```python
from build123d import *

# Parameters (mm, degrees)
SKETCH1_W                = 42.4
SKETCH1_H                = 42.4
BOSS_EXTRUDE1_DEPTH      = 5
BOSS_EXTRUDE2_DEPTH      = 5
BOSS_EXTRUDE2_DEPTH_BACK = 5
SKETCH3_W                = 2.630753666
SKETCH3_H                = 21.2
SKETCH3_W_2              = 21.2
SKETCH3_H_2              = 2.630753666
BOSS_EXTRUDE3_DEPTH      = 12


with BuildPart() as part:
    # Sketch1 → Boss-Extrude1 (new body)
    with BuildSketch(Plane(origin=(0, 0, 0), x_dir=(1, 0, 0), z_dir=(0, 1, 0))):
        with Locations((21.2, 21.2)):
            Rectangle(SKETCH1_W, SKETCH1_H)
    extrude(amount=BOSS_EXTRUDE1_DEPTH)

    # Sketch3 → Boss-Extrude2 (add, two sides: drawn at the far end of the back side and taken through both)
    with BuildSketch(Plane(origin=(0, 5, 0), x_dir=(1, 0, 0), z_dir=(0, 1, 0)).offset(-BOSS_EXTRUDE2_DEPTH_BACK)):
        with Locations((43.715376833, 21.2)):
            Rectangle(SKETCH3_W, SKETCH3_H)
        with Locations((21.2, 43.715376833)):
            Rectangle(SKETCH3_W_2, SKETCH3_H_2)
        with Locations((21.2, -1.315376833)):
            Rectangle(SKETCH3_W_2, SKETCH3_H_2)
        with Locations((-1.315376833, 21.2)):
            Rectangle(SKETCH3_W, SKETCH3_H)
    extrude(amount=BOSS_EXTRUDE2_DEPTH + BOSS_EXTRUDE2_DEPTH_BACK)

    # Sketch4 → Boss-Extrude3 (add)
    with BuildSketch(Plane.XZ):
        Polygon((32.7, -8.601923789), (29.7, -8.601923789), (28.2, -11.2), (29.7, -13.798076211), (32.7, -13.798076211), (34.2, -11.2), align=None)
        Polygon((9.7, -8.601923789), (8.2, -11.2), (9.7, -13.798076211), (12.7, -13.798076211), (14.2, -11.2), (12.7, -8.601923789), align=None)
        Polygon((32.7, -28.601923789), (29.7, -28.601923789), (28.2, -31.2), (29.7, -33.798076211), (32.7, -33.798076211), (34.2, -31.2), align=None)
        Polygon((12.7, -28.601923789), (9.7, -28.601923789), (8.2, -31.2), (9.7, -33.798076211), (12.7, -33.798076211), (14.2, -31.2), align=None)
    extrude(amount=BOSS_EXTRUDE3_DEPTH)


solid = part.part
```
Geometry: final body of the model. Coordinates: model frame, mm. A direction names the side the tool comes from. Give positions to 0.01 mm unless a question says otherwise; leave off trailing zeros. Loops run counter-clockwise (first coordinate to the right, second up) from the corner with the lowest first, then second, coordinate; pieces in that order, holes last. Notation, with made-up numbers: (-11, 33) - (6, 33) arc R23 cw to (6, 41) - close; hole circle Ø1 at (40, 88). An arc over 180 degrees is marked (long way). Answer as CSV lines item,"result". Start each with the question number.
(1) Reachability of faces 1 (the face through (11, -6, -33.798)), 2 (the face through (42.4, 2, -5)), 3 (the face through (21, 7, -42.4)), 4 (the face through (31, -6, -28.602)) from +Z, -Z, +X, -X, +Y, -Y: full face, straight path, thin tool, end or side. Return the list, or none.
(2) Pin query (flat end, axial travel): P1, Ø12, axis at y = -6.5, z = -31, coming from the +X side; P2, Ø2, axis at x = -0.5, y = 5.5, coming from the +Z side; P3, Ø2, axis at x = 7, y = -9.5, coming from the -Z side; P4, Ø0.8, axis at y = 5, z = -43.5, coming from the -X side. Return the tip coordinate at first contact, or that it passes through.
(3) Section query C-C (y = 3.5). Output: boundary loops of the cut face in (x, z).
(4) Section query B-B (z = -26). Output: boundary loops of the cut face in (x, y), and give its area (3 significant figures).
(5) Section query A-A (y = -9.25). Output: boundary loops of the cut face in (x, z).
(6) Section query D-D (x = 15). Output: boundary loops of the cut face in (y, z), and give its area (3 significant figures).
(7) Ray query, line 1 along X through (y, z) = (8, -12.5); line 2 along Y through (x, z) = (10.5, -15.5); line 3 along X through (y, z) = (-7, -32.5). Return the intervals inside material, ascending. Write a range as [from, to].
(8) Mould query, pull axis Z, two halves, no side actions, for faces 5 (the face through (28.96, -5.92, -29.88)), 6 (the face through (45.031, 5, -21)), 7 (the face through (33.44, -5.92, -32.52)). Classes: +Z half, -Z half, draft (parallel to the pull), parting line (faces both ways), or undercut.
Worked answers:
1,face 1,"-Z, +X, -X, -Y"
1,face 2,"+Z, +X, +Y, -Y"
1,face 3,"+X, -X, +Y"
1,face 4,"+X, -X, -Y"
2,P1,"stops at x = 34.2"
2,P2,"stops at z = 0"
2,P3,"passes through"
2,P4,"stops at x = 10.6"
3,outline,"(-2.63, -31.8) - (0, -31.8) - (0, -42.4) - (10.6, -42.4) - (10.6, -45.03) - (31.8, -45.03) - (31.8, -42.4) - (42.4, -42.4) - (42.4, -31.8) - (45.03, -31.8) - (45.03, -10.6) - (42.4, -10.6) - (42.4, 0) - (31.8, 0) - (31.8, 2.63) - (10.6, 2.63) - (10.6, 0) - (0, 0) - (0, -10.6) - (-2.63, -10.6) - close"
4,outline,"(-2.63, 0) - (45.03, 0) - (45.03, 10) - (42.4, 10) - (42.4, 5) - (0, 5) - (0, 10) - (-2.63, 10) - close"
4,area,"265 mm^2"
5,outline,"(8.2, -31.2) - (9.7, -33.8) - (12.7, -33.8) - (14.2, -31.2) - (12.7, -28.6) - (9.7, -28.6) - close; (8.2, -11.2) - (9.7, -13.8) - (12.7, -13.8) - (14.2, -11.2) - (12.7, -8.6) - (9.7, -8.6) - close; (28.2, -31.2) - (29.7, -33.8) - (32.7, -33.8) - (34.2, -31.2) - (32.7, -28.6) - (29.7, -28.6) - close; (28.2, -11.2) - (29.7, -13.8) - (32.7, -13.8) - (34.2, -11.2) - (32.7, -8.6) - (29.7, -8.6) - close"
6,outline,"(0, -45.03) - (10, -45.03) - (10, -42.4) - (5, -42.4) - (5, 0) - (10, 0) - (10, 2.63) - (0, 2.63) - close"
6,area,"265 mm^2"
7,line 1,"x = [-2.63, 0], [42.4, 45.03]"
7,line 2,"y = [0, 5]"
7,line 3,"x = [8.95, 13.45], [28.95, 33.45]"
8,face 5,"undercut"
8,face 6,"draft"
8,face 7,"-Z half"
